from build123d import *

# Parameters (mm, degrees)
SKETCH1_R                                        = 45.466
BOSS_EXTRUDE1_DEPTH                              = 25.4
CSK_FOR_1_4_FLAT_HEAD_MACHINE_SCREW1_D           = 6.5278
CSK_FOR_1_4_FLAT_HEAD_MACHINE_SCREW1_DEPTH       = 25.4
CSK_FOR_1_4_FLAT_HEAD_MACHINE_SCREW1_CSINK_D     = 12.8778
CSK_FOR_1_4_FLAT_HEAD_MACHINE_SCREW1_CSINK_ANGLE = 82
CSK_FOR_1_4_FLAT_HEAD_MACHINE_SCREW1_TIP         = 1.961148974
SKETCH9_R                                        = 53.031918303
CUT_EXTRUDE3_DEPTH                               = 12.7
SKETCH11_R                                       = 48.963999794
CUT_EXTRUDE4_DEPTH                               = 6.35
SKETCH13_R                                       = 45.466
SKETCH13_R_2                                     = 29.398178488
BOSS_EXTRUDE2_DEPTH                              = 3.81
SKETCH12_R                                       = 3.130864452
CUT_EXTRUDE5_DEPTH                               = 6.35
FILLET1_R                                        = 2.54


with BuildPart() as part:
    # Sketch1 → Boss-Extrude1 (new body)
    with BuildSketch(Plane(origin=(0, 0, 0), x_dir=(1, 0, 0), z_dir=(0, 1, 0))):
        Circle(SKETCH1_R)
    extrude(amount=BOSS_EXTRUDE1_DEPTH)

    # CSK for 1/4 Flat Head Machine Screw1
    with Locations(Plane(origin=(0, 25.4, 0), x_dir=(1, 0, 0), z_dir=(0, 1, 0))):
        with Locations((0, 0)):
            CounterSinkHole(CSK_FOR_1_4_FLAT_HEAD_MACHINE_SCREW1_D / 2, CSK_FOR_1_4_FLAT_HEAD_MACHINE_SCREW1_CSINK_D / 2, depth=CSK_FOR_1_4_FLAT_HEAD_MACHINE_SCREW1_DEPTH, counter_sink_angle=CSK_FOR_1_4_FLAT_HEAD_MACHINE_SCREW1_CSINK_ANGLE)
            with Locations((0, 0, -(CSK_FOR_1_4_FLAT_HEAD_MACHINE_SCREW1_DEPTH + CSK_FOR_1_4_FLAT_HEAD_MACHINE_SCREW1_TIP / 2))):  # 118° drill point
                Cone(0, CSK_FOR_1_4_FLAT_HEAD_MACHINE_SCREW1_D / 2, CSK_FOR_1_4_FLAT_HEAD_MACHINE_SCREW1_TIP, mode=Mode.SUBTRACT)

    # Sketch9 → Cut-Extrude3 (cut)
    with BuildSketch(Plane.XZ):
        Circle(SKETCH9_R)
    extrude(amount=-CUT_EXTRUDE3_DEPTH, mode=Mode.SUBTRACT)

    # Sketch11 → Cut-Extrude4 (cut)
    with BuildSketch(Plane.XZ.offset(-12.7)):
        Circle(SKETCH11_R)
    extrude(amount=-CUT_EXTRUDE4_DEPTH, mode=Mode.SUBTRACT)

    # Sketch13 → Boss-Extrude2 (add)
    with BuildSketch(Plane(origin=(0, 25.4, 0), x_dir=(1, 0, 0), z_dir=(0, 1, 0))):
        Circle(SKETCH13_R)
        Circle(SKETCH13_R_2, mode=Mode.SUBTRACT)
    extrude(amount=BOSS_EXTRUDE2_DEPTH)

    # Sketch12 → Cut-Extrude5 (cut)
    with BuildSketch(Plane.XZ.offset(-19.05)):
        with Locations((0, 38.309864452)):
            Circle(SKETCH12_R)
        with Locations((9.915322535, 37.004487476)):
            Circle(SKETCH12_R)
        with Locations((19.154932226, 33.177315831)):
            Circle(SKETCH12_R)
        with Locations((27.08916494, 27.08916494)):
            Circle(SKETCH12_R)
        with Locations((33.177315831, 19.154932226)):
            Circle(SKETCH12_R)
        with Locations((37.004487476, 9.915322535)):
            Circle(SKETCH12_R)
        with Locations((38.309864452, 0)):
            Circle(SKETCH12_R)
        with Locations((37.004487476, -9.915322535)):
            Circle(SKETCH12_R)
        with Locations((33.177315831, -19.154932226)):
            Circle(SKETCH12_R)
        with Locations((27.08916494, -27.08916494)):
            Circle(SKETCH12_R)
        with Locations((19.154932226, -33.177315831)):
            Circle(SKETCH12_R)
        with Locations((9.915322535, -37.004487476)):
            Circle(SKETCH12_R)
        with Locations((0, -38.309864452)):
            Circle(SKETCH12_R)
        with Locations((-9.915322535, -37.004487476)):
            Circle(SKETCH12_R)
        with Locations((-19.154932226, -33.177315831)):
            Circle(SKETCH12_R)
        with Locations((-27.08916494, -27.08916494)):
            Circle(SKETCH12_R)
        with Locations((-33.177315831, -19.154932226)):
            Circle(SKETCH12_R)
        with Locations((-37.004487476, -9.915322535)):
            Circle(SKETCH12_R)
        with Locations((-38.309864452, 0)):
            Circle(SKETCH12_R)
        with Locations((-37.004487476, 9.915322535)):
            Circle(SKETCH12_R)
        with Locations((-33.177315831, 19.154932226)):
            Circle(SKETCH12_R)
        with Locations((-27.08916494, 27.08916494)):
            Circle(SKETCH12_R)
        with Locations((-19.154932226, 33.177315831)):
            Circle(SKETCH12_R)
        with Locations((-9.915322535, 37.004487476)):
            Circle(SKETCH12_R)
    extrude(amount=-CUT_EXTRUDE5_DEPTH, mode=Mode.SUBTRACT)

    # Fillet1
    fillet1_edges = [part.edges().sort_by_distance(p)[0] for p in [
        (-45.466, 29.21, 0),
        (-29.398178488, 29.21, 0),
    ]]
    fillet(fillet1_edges, radius=FILLET1_R)


solid = part.part
The model under review builds one solid part; all positions refer to its coordinate system, in mm. A direction names the side the tool comes from. Give positions to 0.01 mm unless a question says otherwise; leave off trailing zeros. Loops run counter-clockwise (first coordinate to the right, second up) from the corner with the lowest first, then second, coordinate; pieces in that order, holes last. Notation, with made-up numbers: (56.25, -20) -> (112.25, -20) arc R13 ccw to (112.25, 0) -> close; hole circle Ø1 at (4, 10.25). An arc over 180 degrees is marked (long way). Put each result on its own line as item: value. Start each with the question number.
1. Wall thickness on probe 1 along X at (y, z) = (21.75, 28.5); probe 2 along Z at (x, y) = (11, 21.5): over which ranges is each line inside the solid? List them lowest first.
2. We need section A-A on z = 0. State the section outline as (x, y) points.
3. Mouldability with a two-part tool opening along X and no side actions: class faces 1 (the face through (33, 25.4, -19)), 2 (the face through (-32, 29.21, 3)) as released by +X, released by -X, zero draft, split by the parting line, or undercut.
4. We need section B-B on x = 0. State the section outline as (y, z) points.
5. We need section C-C on y = 28. State the section outline as (x, z) points.
6. Clearance check with flat-ended pins moving along their axes: P1, Ø1.9, axis at x = 9, z = 38.5, coming from the -Y side; P2, Ø6, axis at x = 6.5, y = 25, coming from the +Z side; P3, Ø2, axis at y = 25, z = -32.5, coming from the -X side. State where each tip first meets the part, or that it passes through.
7. For faces 3 (the face through (0, 25.4, -7)), 4 (the face through (0.708, 20.38, 3.186)), 5 (the face through (-33, 25.4, 19)), list the 3-axis set-ups (+Z, -Z, +X, -X, +Y, -Y) from which the entire face can be reached by the end or side of a thin tool; tool diameter is ignored.
Determined:
1. probe 1: -35.42 to -29.88, -24.29 to 24.29, 29.88 to 35.42
1. probe 2: -44.12 to -39.94, -34.07 to 34.07, 39.94 to 44.12
2. outline: (-45.47, 19.05) -> (-41.44, 19.05) -> (-41.44, 25.4) -> (-35.18, 25.4) -> (-35.18, 19.05) -> (-3.26, 19.05) -> (-3.26, 21.75) -> (-6.44, 25.4) -> (-29.4, 25.4) -> (-29.4, 26.67) arc R2.54 ccw to (-31.94, 29.21) -> (-42.93, 29.21) arc R2.54 ccw to (-45.47, 26.67) -> close; (3.26, 19.05) -> (35.18, 19.05) -> (35.18, 25.4) -> (41.44, 25.4) -> (41.44, 19.05) -> (45.47, 19.05) -> (45.47, 26.67) arc R2.54 ccw to (42.93, 29.21) -> (31.94, 29.21) arc R2.54 ccw to (29.4, 26.67) -> (29.4, 25.4) -> (6.44, 25.4) -> (3.26, 21.75) -> close
3. face 1: undercut
3. face 2: zero draft
4. outline: (19.05, -45.47) -> (26.67, -45.47) arc R2.54 ccw to (29.21, -42.93) -> (29.21, -31.94) arc R2.54 ccw to (26.67, -29.4) -> (25.4, -29.4) -> (25.4, -6.44) -> (21.75, -3.26) -> (19.05, -3.26) -> (19.05, -35.18) -> (25.4, -35.18) -> (25.4, -41.44) -> (19.05, -41.44) -> close; (19.05, 3.26) -> (21.75, 3.26) -> (25.4, 6.44) -> (25.4, 29.4) -> (26.67, 29.4) arc R2.54 ccw to (29.21, 31.94) -> (29.21, 42.93) arc R2.54 ccw to (26.67, 45.47) -> (19.05, 45.47) -> (19.05, 41.44) -> (25.4, 41.44) -> (25.4, 35.18) -> (19.05, 35.18) -> close
5. outline: circle Ø90.18 at (0, 0); hole circle Ø59.55 at (0, 0)
6. P1: y = 25.4
6. P2: z = 45.33
6. P3: x = -32.79
7. face 3: +Y
7. face 4: +Y, -Y
7. face 5: -Y
